For this review, take the finished solid that the model builds, in its own axes (mm). Face numbers are marked on the shaded views. A direction names the side the tool comes from. Give positions to 0.01 mm unless a question says otherwise; leave off trailing zeros. Order: outer loops, then holes, each group sorted by start corner. A loop starts at its lowest first (then second) coordinate and runs counter-clockwise, first axis right, second up. Notation, with made-up numbers: (56.5, 40.25) - (90.5, 40.25) arc R17 ccw to (90.5, 52.25) - close; hole circle Ø6 at (77, 57). An arc over 180 degrees is marked (long way). Put each result on its own line as item: value. Start each with the question number.
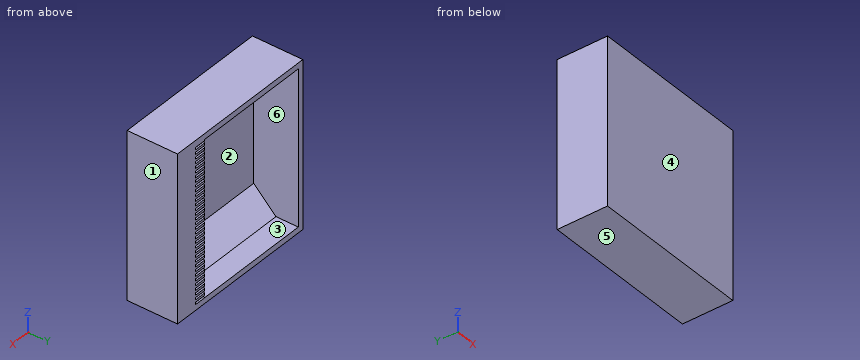
```python
from build123d import *

# Parameters (mm, degrees)
SKETCH_1_W                 = 145
SKETCH_1_H                 = 44
EXTRUDE_1_DEPTH            = 139
SHELL_1_T                  = -5
SHELL_1_THICKNESS_2_FACE_W = 135
SHELL_1_THICKNESS_2_FACE_H = 39
SHELL_1_THICKNESS_2_DEPTH  = 25
EXTRUDE_2_REACH            = 204.28
CUT_EXTRUDE_START          = -10
CUT_EXTRUDE_1_DEPTH        = 10
PATTERN_LINEAR_2_COUNT     = 34
PATTERN_LINEAR_2_PITCH     = 4


with BuildPart() as part:
    # 스케치1 → 보스-돌출1 (new body)
    with BuildSketch(Plane(origin=(0, 0, 0), x_dir=(0, 0, -1), z_dir=(1, 0, 0))):
        with Locations((-72.5, 22)):
            Rectangle(SKETCH_1_W, SKETCH_1_H)
    extrude(amount=EXTRUDE_1_DEPTH)

    # 쉘1
    shell_1_openings = [part.faces().sort_by_distance(p)[0] for p in [
        (69.5, 44, 72.5),
    ]]
    offset(amount=SHELL_1_T, openings=shell_1_openings, kind=Kind.INTERSECTION)

    # 쉘1 thickness 2 face (on inner face of the shell) → 쉘1 thickness 2 (add)
    with BuildSketch(Plane(origin=(134, 24.5, 72.5), x_dir=(0, 0, 1), z_dir=(1, 0, 0))):
        Rectangle(SHELL_1_THICKNESS_2_FACE_W, SHELL_1_THICKNESS_2_FACE_H)
    extrude(amount=-SHELL_1_THICKNESS_2_DEPTH)

    # 스케치3 → 보스-돌출2 (add, up to next)
    with BuildSketch(Plane(origin=(5, 0, 0), x_dir=(0, 0, -1), z_dir=(1, 0, 0)), mode=Mode.PRIVATE) as extrude_2_sk1:
        Polygon((-5, 24.5), (-24.5, 5), (-5, 5), align=None)
    extrude_2_tool1 = extrude(extrude_2_sk1.sketch, amount=EXTRUDE_2_REACH, mode=Mode.PRIVATE) - part.part
    add(extrude_2_tool1.solids().sort_by_distance((5, 11.5, 11.5))[0])

    # 스케치4 → 컷-돌출1 (cut)
    with BuildSketch(Plane.ZY.offset(-109).offset(CUT_EXTRUDE_START)):
        with BuildLine():
            Line((4.168052643, 46.265280356), (7.789262128, 46.265280356))
            ThreePointArc((7.789262128, 46.265280356), (7.302805176, 44.485235891), (5.978657386, 43.2))
            ThreePointArc((5.978657386, 43.2), (4.654509595, 44.485235891), (4.168052643, 46.265280356))
        make_face()
    cut_extrude_1 = extrude(amount=CUT_EXTRUDE_1_DEPTH, mode=Mode.SUBTRACT)

    # 선형 패턴2: 컷-돌출1 ×34
    with Locations(*[(0, 0, i * PATTERN_LINEAR_2_PITCH) for i in range(1, PATTERN_LINEAR_2_COUNT)]):
        add(cut_extrude_1, mode=Mode.SUBTRACT)


solid = part.part
```
1. The part is to be moulded in two halves that separate along X. For the marked faces 1, 2, 3 and 4, say which applies: released by +X, released by -X, zero draft, split by the parting line, or undercut.
2. Add section C-C, the plane y = 27. Give the boundary of the cut face in (x, z).
3. Tool access review of the marked faces 5 and 6: name each direction out of +Z, -Z, +X, -X, +Y, -Y from which nothing blocks a thin tool from reaching the whole face with its end or side.
4. Add section A-A, the plane x = 29. Give the boundary of the cut face in (y, z), then the cut area to 3 significant figures.
5. Add section B-B, the plane y = 15. Give the boundary of the cut face in (x, z).
6. Clearance check with a flat-ended pin moving along its axis: pin 1 (4 mm diameter, centred on x = 53, z = 72.5, fed in from +Y). State where the tip first meets the part, or that it passes through.
7. Wall thickness on line 1 (X direction, y = 18.5, z = 103.5); line 2 (Z direction, x = 20, y = 30); line 3 (Y direction, x = 14, z = 28): over which ranges is each line inside the solid? List them lowest first. Write a range as from..to.
Found:
1. face 1: released by +X
1. face 2: undercut
1. face 3: undercut
1. face 4: zero draft
2. outline: (0, 0) - (139, 0) - (139, 145) - (0, 145) - close; hole (5, 5) - (109, 5) - (109, 140) - (5, 140) - close
3. face 5: -Z, +X, -X, +Y, -Y
3. face 6: +Y
4. outline: (0, 0) - (44, 0) - (44, 5) - (24.5, 5) - (5, 24.5) - (5, 140) - (44, 140) - (44, 145) - (0, 145) - close
4. area: 1,310 mm^2
5. outline: (0, 0) - (139, 0) - (139, 145) - (0, 145) - close; hole (5, 14.5) - (109, 14.5) - (109, 140) - (5, 140) - close
6. pin 1: stops at y = 5
7. line 1: x = 0..5, 109..139
7. line 2: z = 0..5, 140..145
7. line 3: y = 0..5
